from build123d import *

# Parameters (mm, degrees)
SKETCH1_W            = 26
SKETCH1_H            = 26
SKETCH1_W_2          = 22
SKETCH1_H_2          = 22
BOSS_EXTRUDE16_DEPTH = 8
SKETCH1_5_W          = 22
SKETCH1_5_H          = 22
BOSS_EXTRUDE17_DEPTH = 2
SKETCH4_W            = 4.2
SKETCH4_H            = 4.2
CUT_EXTRUDE3_DEPTH   = 1.2
SKETCH8_W            = 3.8
SKETCH8_H            = 3.8
CUT_EXTRUDE4_DEPTH   = 2
HOLE2_START          = -13
HOLE2_OUTLINE_R      = 1.55
HOLE2_DEPTH          = 26
HOLE4_START          = -13
HOLE4_OUTLINE_R      = 1
HOLE4_DEPTH          = 2
SKETCH15_W           = 3.4
SKETCH15_H           = 3.4
CUT_EXTRUDE25_DEPTH  = 2
SKETCH15_6_W         = 3.8
SKETCH15_6_H         = 3.8
SKETCH15_6_W_2       = 3.4
SKETCH15_6_H_2       = 3.4
CUT_EXTRUDE26_DEPTH  = 1.2


# Read off the part's stored shape, not the designer's step: Hole2, Hole4
with BuildPart() as part:
    # Sketch1 → Boss-Extrude16 (new body)
    with BuildSketch(Plane.XY):
        Rectangle(SKETCH1_W, SKETCH1_H)
        Rectangle(SKETCH1_W_2, SKETCH1_H_2, mode=Mode.SUBTRACT)
    extrude(amount=BOSS_EXTRUDE16_DEPTH)

    # Sketch1<5> → Boss-Extrude17 (add)
    with BuildSketch(Plane.XY):
        Rectangle(SKETCH1_5_W, SKETCH1_5_H)
    extrude(amount=BOSS_EXTRUDE17_DEPTH)

    # Sketch4 → Cut-Extrude3 (cut)
    with BuildSketch(Plane.XY):
        Rectangle(SKETCH4_W, SKETCH4_H)
    extrude(amount=CUT_EXTRUDE3_DEPTH, mode=Mode.SUBTRACT)

    # Sketch8 → Cut-Extrude4 (cut)
    with BuildSketch(Plane(origin=(0, 0, 1.2), x_dir=(-1, 0, 0), z_dir=(0, 0, -1))):
        Rectangle(SKETCH8_W, SKETCH8_H)
    extrude(amount=-CUT_EXTRUDE4_DEPTH, mode=Mode.SUBTRACT)

    # Hole2 outline → Hole2 (cut)
    with BuildSketch(Plane(origin=(0, 0, 0), x_dir=(1, 0, 0), z_dir=(0, 1, 0)).offset(HOLE2_START)):
        with Locations((-0.00435538, -3.992237836)):
            Circle(HOLE2_OUTLINE_R)
    extrude(amount=HOLE2_DEPTH, mode=Mode.SUBTRACT)

    # Hole4 outline → Hole4 (cut)
    with BuildSketch(Plane.YZ.offset(HOLE4_START)):
        with Locations((0.004397166, 4.002298356)):
            Circle(HOLE4_OUTLINE_R)
    extrude(amount=HOLE4_DEPTH, mode=Mode.SUBTRACT)

    # Sketch15 → Cut-Extrude25 (cut)
    with BuildSketch(Plane(origin=(13, 0, 0), x_dir=(0, 0, -1), z_dir=(1, 0, 0))):
        with Locations((-4, 0)):
            Rectangle(SKETCH15_W, SKETCH15_H)
    extrude(amount=-CUT_EXTRUDE25_DEPTH, mode=Mode.SUBTRACT)

    # Sketch15<6> → Cut-Extrude26 (cut)
    with BuildSketch(Plane(origin=(13, 0, 0), x_dir=(0, 0, -1), z_dir=(1, 0, 0))):
        with Locations((-4, 0)):
            Rectangle(SKETCH15_6_W, SKETCH15_6_H)
        with Locations((-4, 0)):
            Rectangle(SKETCH15_6_W_2, SKETCH15_6_H_2, mode=Mode.SUBTRACT)
    extrude(amount=-CUT_EXTRUDE26_DEPTH, mode=Mode.SUBTRACT)


solid = part.part
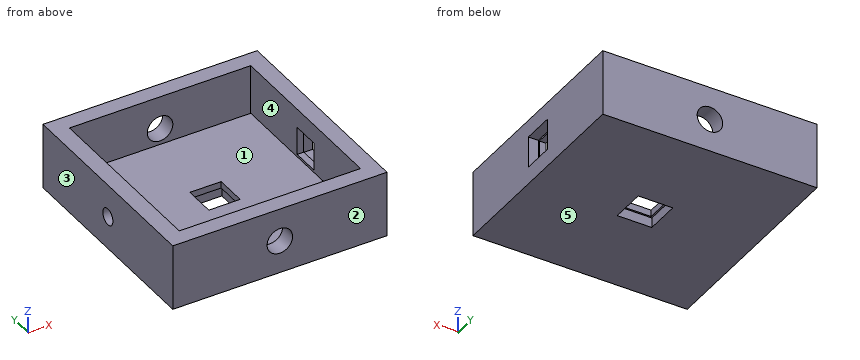
Input: part model. Units: mm. Frame: model coordinates. Face numbers are marked on the shaded views. A direction names the side the tool comes from. Round coordinates to 2 decimals unless told otherwise and drop trailing zeros. Loops run counter-clockwise (first coordinate to the right, second up) from the corner with the lowest first, then second, coordinate; pieces in that order, holes last. Notation, with made-up numbers: M 23.25,50 L 55.25,50 A11 cw 55.25,59 Z; hole C 31.25,40.5 d2. An arc over 180 degrees is marked long. Answer as CSV lines item,"result". Start each with the question number.
(1) Section A-A, the plane x = -4. Output: boundary loops of the cut face in (y, z), plus the area to 3 significant figures.
(2) Section C-C, the plane z = 6.25. Output: boundary loops of the cut face in (x, y), plus the area to 3 significant figures.
(3) Line query: line 1 (Y direction, x = -1.75, z = 1.25); line 2 (X direction, y = -3.5, z = 5). Output: solid intervals per line, ascending. Write a range as [from, to].
(4) First-contact query: pin 1 (12 mm diameter, centred on x = -2.5, y = -1.5, fed in from -Z). Flat tip, straight axial feed; report the tip coordinate or a pass-through.
(5) Reachability of the marked faces 1 and 2 from +Z, -Z, +X, -X, +Y, -Y: full face, straight path, thin tool, end or side. Return the list, or none.
(6) Section D-D, the plane z = 3.5. Output: boundary loops of the cut face in (x, y), plus the area to 3 significant figures.
(7) Draft query along X for the marked faces 3, 4 and 5. Return one class per face: released by +X, released by -X, zero draft, split by the parting line, or undercut.
Values found:
1,outline,"M -13,0 L 13,0 L 13,8 L 11,8 L 11,2 L -11,2 L -11,8 L -13,8 Z"
1,area,"76.0 mm²"
2,outline,"M -13,-13 L 13,-13 L 13,13 L -13,13 Z; hole M -11,-11 L 11,-11 L 11,11 L -11,11 Z"
2,area,"192 mm²"
3,line 1,"y = [-13, -1.9], [1.9, 13]"
3,line 2,"x = [-13, -11], [11, 13]"
4,pin 1,"stops at z = 0"
5,face 1,"+Z"
5,face 2,"+Z, -Z, +X, -X, -Y"
6,outline,"M -13,-13 L -1.47,-13 L -1.47,-11 L -11,-11 L -11,-0.86 L -13,-0.86 Z; M -13,0.87 L -11,0.87 L -11,11 L -1.47,11 L -1.47,13 L -13,13 Z; M 1.47,-13 L 13,-13 L 13,-1.9 L 11.8,-1.9 L 11.8,-1.7 L 11,-1.7 L 11,-11 L 1.47,-11 Z; M 1.47,11 L 11,11 L 11,1.7 L 11.8,1.7 L 11.8,1.9 L 13,1.9 L 13,13 L 1.47,13 Z"
6,area,"170 mm²"
7,face 3,"released by -X"
7,face 4,"undercut"
7,face 5,"zero draft"
